from build123d import *

# Parameters (mm, degrees)
BOSS_EXTRUDE1_DEPTH      = 75
BOSS_EXTRUDE1_DEPTH_BACK = 75
SKETCH1_W                = 40
SKETCH1_H                = 30
SKETCH3_R                = 3.1
CUT_EXTRUDE1_DEPTH       = 150
CUT_EXTRUDE2_DEPTH       = 150
CUT_EXTRUDE2_DEPTH_BACK  = 150
SKETCH4_W                = 22.5
SKETCH4_H                = 22.5
SKETCH7_W                = 58.590655802
SKETCH7_H                = 20
CUT_EXTRUDE5_DEPTH       = 40
SKETCH8_W                = 20
SKETCH8_H                = 35
CUT_EXTRUDE6_DEPTH       = 35
FILLET2_R                = 0.5
FILLET3_R                = 0.5
CUT_EXTRUDE7_DEPTH       = 102
CUT_EXTRUDE7_DEPTH_BACK  = 10
SKETCH6_R                = 1.5


with BuildPart() as part:
    # Sketch1 → Boss-Extrude1 (new, two sides: drawn at the far end of the back side and taken through both)
    with BuildSketch(Plane(origin=(0, 0, 0), x_dir=(1, 0, 0), z_dir=(0, 1, 0)).offset(-BOSS_EXTRUDE1_DEPTH_BACK)):
        Rectangle(SKETCH1_W, SKETCH1_H)
    extrude(amount=BOSS_EXTRUDE1_DEPTH + BOSS_EXTRUDE1_DEPTH_BACK)

    # Sketch3 → Cut-Extrude1 (cut)
    with BuildSketch(Plane(origin=(20, 0, 0), x_dir=(0, 0, -1), z_dir=(1, 0, 0))):
        with Locations((0, 30)):
            Circle(SKETCH3_R)
    cut_extrude1 = extrude(amount=-CUT_EXTRUDE1_DEPTH, mode=Mode.SUBTRACT)

    # Mirror1: Cut-Extrude1 across plane
    add(cut_extrude1.mirror(Plane.ZX), mode=Mode.SUBTRACT)

    # Sketch4 → Cut-Extrude2 (cut, two sides: drawn at the far end of the back side and taken through both)
    with BuildSketch(Plane(origin=(0, 0, 0), x_dir=(0, 0, -1), z_dir=(1, 0, 0)).offset(-CUT_EXTRUDE2_DEPTH_BACK)):
        Rectangle(SKETCH4_W, SKETCH4_H)
    extrude(amount=CUT_EXTRUDE2_DEPTH + CUT_EXTRUDE2_DEPTH_BACK, mode=Mode.SUBTRACT)

    # Sketch7 → Cut-Extrude5 (cut)
    with BuildSketch(Plane(origin=(0, 75, 0), x_dir=(1, 0, 0), z_dir=(0, 1, 0))):
        with Locations((14.295327901, 0)):
            Rectangle(SKETCH7_W, SKETCH7_H)
    extrude(amount=-CUT_EXTRUDE5_DEPTH, mode=Mode.SUBTRACT)

    # Sketch8 → Cut-Extrude6 (cut)
    with BuildSketch(Plane(origin=(20, 0, 0), x_dir=(0, 0, -1), z_dir=(1, 0, 0))):
        with Locations((0, -52.5)):
            Rectangle(SKETCH8_W, SKETCH8_H)
    extrude(amount=-CUT_EXTRUDE6_DEPTH, mode=Mode.SUBTRACT)

    # Fillet2
    fillet2_edges = [part.edges().sort_by_distance(p)[0] for p in [
        (20, 75, 12.5),
        (0, 75, -15),
        (-20, 75, 0),
        (0, 75, 15),
        (20, 75, -12.5),
        (2.5, 75, -10),
        (2.5, 75, 10),
        (-15, 75, 0),
    ]]
    fillet(fillet2_edges, radius=FILLET2_R)

    # Fillet3
    fillet3_edges = [part.edges().sort_by_distance(p)[0] for p in [
        (20, -52.5, 10),
        (20, -70, 0),
        (20, -52.5, -10),
        (20, -35, 0),
    ]]
    fillet(fillet3_edges, radius=FILLET3_R)

    # Sketch6 → Cut-Extrude7 (cut, two sides: drawn at the far end of the back side and taken through both)
    with BuildSketch(Plane(origin=(0, 0, 11.25), x_dir=(-1, 0, 0), z_dir=(0, 0, -1)).offset(-CUT_EXTRUDE7_DEPTH_BACK)):
        with Locations(Location((0, 0, 0), (0, 0, 180))):
            Circle(SKETCH6_R)
    extrude(amount=CUT_EXTRUDE7_DEPTH + CUT_EXTRUDE7_DEPTH_BACK, mode=Mode.SUBTRACT)


solid = part.part
Model file for the job. Use its own axes, mm. A direction names the side the tool comes from. Coordinates: 2 decimals unless noted, no trailing zeros. Order: outer loops, then holes, each group sorted by start corner. A loop starts at its lowest first (then second) coordinate and runs counter-clockwise, first axis right, second up. Notation, with made-up numbers: M -7.75,55 L 45.25,55 A32 ccw 45.25,94 Z; hole C -35.75,83.25 d11. An arc over 180 degrees is marked long. Return JSON: item names as keys, results as strings.
1. Saw through at D-D (y = 30). Give the cut face in (x, z), and give its area (3 significant figures).
Ans:
{"outline": "M -20,-15 L 20,-15 L 20,-3.1 L -20,-3.1 Z; M -20,3.1 L 20,3.1 L 20,15 L -20,15 Z", "area": "952 mm^2"}
2. Tool access for faces 4 (the face through (0, 2, -11.25)), 5 (the face through (-15, 55, 0)), 6 (the face through (20, 15, 0)), 7 (the face through (2, -70, 0)), 8 (the face through (0, -75, 0)): list every direction of +Z, -Z, +X, -X, +Y, -Y with a clear straight run to the whole face (end or side of a thin tool).
Ans:
{"face 4": "+X, -X", "face 5": "+X, +Y", "face 6": "+Z, -Z, +X, +Y, -Y", "face 7": "+X", "face 8": "+Z, -Z, +X, -X, -Y"}
3. Saw through at C-C (z = 8). Give the cut face in (x, y).
Ans:
{"outline": "M -20,-75 L 20,-75 L 20,-70.5 A0.5 ccw 19.5,-70 L -15,-70 L -15,-35 L 19.5,-35 A0.5 ccw 20,-34.5 L 20,-11.25 L -20,-11.25 Z; M -20,11.25 L 20,11.25 L 20,35 L -15,35 L -15,74.5 A0.5 ccw -15.5,75 L -19.5,75 A0.5 ccw -20,74.5 Z"}
4. Saw through at A-A (x = 0). Give the number of separate pieces and of enclosed holes in the cut face, and give its area (3 significant figures).
Ans:
{"separate pieces": "2", "enclosed holes": "3", "area": "2,410 mm^2"}
5. Saw through at B-B (y = 0). Give the cut face in (x, z), and give its area (4 significant figures).
Ans:
{"outline": "M -20,-15 L -1.5,-15 L -1.5,-11.25 L -20,-11.25 Z; M -20,11.25 L -1.5,11.25 L -1.5,15 L -20,15 Z; M 1.5,-15 L 20,-15 L 20,-11.25 L 1.5,-11.25 Z; M 1.5,11.25 L 20,11.25 L 20,15 L 1.5,15 Z", "area": "277.5 mm^2"}
6. Flat gauge pins, fed straight in: pin 1 (8 mm diameter, centred on y = -30, z = 0, fed in from +X); pin 2 (3 mm diameter, centred on y = -49, z = -6, fed in from +X); pin 3 (8 mm diameter, centred on x = 1.5, z = -2.5, fed in from +Y). Where does each tip first touch, or does it go through?
Ans:
{"pin 1": "x = 20", "pin 2": "x = -15", "pin 3": "y = 35"}
7. Pull direction Y, two halves, no side cores. Call faces 1 (the face through (-4, 75, 11)), 2 (the face through (-20, -1, 14)), 3 (the face through (0.28, 33.074, 0.404)): +Y half, -Y half, draft (parallel to the pull), parting line (faces both ways), or undercut.
Ans:
{"face 1": "+Y half", "face 2": "draft", "face 3": "undercut"}
8. Drill centre lines: probe 1 along Y at (x, z) = (-8.5, 0); probe 2 along Y at (x, z) = (-6, 6); probe 3 along Z at (x, y) = (11.5, 48). Where is each one in solid material? Low to high.
Ans:
{"probe 1": "-75 to -70, -35 to -33.1, -26.9 to -11.25, 11.25 to 26.9, 33.1 to 35", "probe 2": "-75 to -70, -35 to -11.25, 11.25 to 35", "probe 3": "-15 to -10, 10 to 15"}
